from build123d import *
from build123d.topology import SkipClean

# Parameters (mm, degrees)
SKETCH1_R           = 7
SKETCH1_R_2         = 5.2
BOSS_EXTRUDE1_DEPTH = 15.66
BOSS_EXTRUDE2_START = -4
SKETCH2_W           = 6
SKETCH2_H           = 4
BOSS_EXTRUDE2_DEPTH = 4
CUT_EXTRUDE2_START  = -2
SKETCH2_3_W         = 6
SKETCH2_3_H         = 4
CUT_EXTRUDE2_DEPTH  = 2
SKETCH4_R           = 1.5
CUT_EXTRUDE1_DEPTH  = 10
FILLET7_R           = 3
BOSS_EXTRUDE3_START = -1
SKETCH5_R           = 5.2
BOSS_EXTRUDE3_DEPTH = 1
CUT_EXTRUDE3_DEPTH  = 15.66
FILLET8_R           = 3
BOSS_EXTRUDE4_DEPTH = 2


with BuildPart() as part:
    # Sketch1 → Boss-Extrude1 (new body)
    with BuildSketch(Plane(origin=(0, 0, 0), x_dir=(1, 0, 0), z_dir=(0, 1, 0))):
        with Locations(Location((0, 0, 0), (0, 0, 270))):
            Circle(SKETCH1_R)
        with Locations(Location((0, 0, 0), (0, 0, 270))):
            Circle(SKETCH1_R_2, mode=Mode.SUBTRACT)
    extrude(amount=BOSS_EXTRUDE1_DEPTH)

    # Sketch2 → Boss-Extrude2 (add)
    with BuildSketch(Plane(origin=(0, 15.66, 0), x_dir=(1, 0, 0), z_dir=(0, 1, 0)).offset(BOSS_EXTRUDE2_START)):
        with Locations((-10.67, -9)):
            Rectangle(SKETCH2_W, SKETCH2_H)
        with BuildLine():
            ThreePointArc((0, -7), (-7, 0), (0, 7))
            Line((0, 7), (-7.67, 7))
            Line((-7.67, 7), (-13.67, 7))
            Line((-13.67, 7), (-13.67, -7))
            Line((-13.67, -7), (-7.67, -7))
            Line((-7.67, -7), (0, -7))
        make_face()
        with Locations((-10.67, 9)):
            Rectangle(SKETCH2_W, SKETCH2_H)
    extrude(amount=BOSS_EXTRUDE2_DEPTH)

    # Sketch2<3> → Cut-Extrude2 (cut)
    with SkipClean():  # the faces are left unmerged after this step: merging them gives an invalid solid
        with BuildSketch(Plane(origin=(0, 15.66, 0), x_dir=(1, 0, 0), z_dir=(0, 1, 0)).offset(CUT_EXTRUDE2_START)):
            with BuildLine():
                ThreePointArc((0, -7), (-7, 0), (0, 7))
                Line((0, 7), (-7.67, 7))
                Line((-7.67, 7), (-13.67, 7))
                Line((-13.67, 7), (-13.67, -7))
                Line((-13.67, -7), (-7.67, -7))
                Line((-7.67, -7), (0, -7))
            make_face()
            with Locations((-10.67, 9)):
                Rectangle(SKETCH2_3_W, SKETCH2_3_H)
            with Locations((-10.67, -9)):
                Rectangle(SKETCH2_3_W, SKETCH2_3_H)
        extrude(amount=CUT_EXTRUDE2_DEPTH, mode=Mode.SUBTRACT)

    # Sketch4 → Cut-Extrude1 (cut)
    with SkipClean():  # the faces are left unmerged after this step: merging them gives an invalid solid
        with BuildSketch(Plane.XZ.offset(-11.66)):
            with Locations(Location((-10.68, -8, 0), (0, 0, 270))):
                Circle(SKETCH4_R)
            with Locations(Location((-10.68, 8, 0), (0, 0, 270))):
                Circle(SKETCH4_R)
        extrude(amount=-CUT_EXTRUDE1_DEPTH, mode=Mode.SUBTRACT)

    # Fillet7
    fillet7_edges = [part.edges().sort_by_distance(p)[0] for p in [
        (-7.67, 12.66, 7),
    ]]
    fillet(fillet7_edges, radius=FILLET7_R)

    # Sketch5 → Boss-Extrude3 (add)
    with SkipClean():  # the faces are left unmerged after this step: merging them gives an invalid solid
        with BuildSketch(Plane(origin=(0, 15.66, 0), x_dir=(1, 0, 0), z_dir=(0, 1, 0)).offset(BOSS_EXTRUDE3_START)):
            with Locations(Location((0, 0, 0), (0, 0, 270))):
                Circle(SKETCH5_R)
        extrude(amount=BOSS_EXTRUDE3_DEPTH)

    # Sketch6 → Cut-Extrude3 (cut)
    with BuildSketch(Plane.XZ):
        with BuildLine():
            Line((6, -3.605551275), (6, 3.605551275))
            ThreePointArc((6, 3.605551275), (7, 0), (6, -3.605551275))
        make_face()
    extrude(amount=-CUT_EXTRUDE3_DEPTH, mode=Mode.SUBTRACT)

    # Fillet8
    fillet8_edges = [part.edges().sort_by_distance(p)[0] for p in [
        (6, 15.66, 0),
    ]]
    fillet(fillet8_edges, radius=FILLET8_R)

    # Sketch7 → Boss-Extrude4 (add)
    with BuildSketch(Plane(origin=(0, 13.66, 0), x_dir=(1, 0, 0), z_dir=(0, 1, 0))):
        with BuildLine():
            Line((-13.67, 4.5), (-13.67, -4.5))
            Line((-13.67, -4.5), (-5.361902647, -4.5))
            ThreePointArc((-5.361902647, -4.5), (-7, 0), (-5.361902647, 4.5))
            Line((-5.361902647, 4.5), (-13.67, 4.5))
        make_face()
    extrude(amount=BOSS_EXTRUDE4_DEPTH)


solid = part.part
The model under review builds one solid part; all positions refer to its coordinate system, in mm. A direction names the side the tool comes from. Give positions to 0.01 mm unless a question says otherwise; leave off trailing zeros. Loops run counter-clockwise (first coordinate to the right, second up) from the corner with the lowest first, then second, coordinate; pieces in that order, holes last. Notation, with made-up numbers: (84, -13) -> (134, -13) arc R17 cw to (134, 5) -> close; hole circle Ø11 at (37, -20.5). An arc over 180 degrees is marked (long way). Put each result on its own line as item: value. Start each with the question number.
1. We need section C-C on y = 14.25. State the section outline as (x, z) points.
2. We need section B-B on z = -8. State the section outline as (x, y) points.
3. Wall thickness on probe 1 along X at (y, z) = (11.25, 0); probe 2 along Z at (x, y) = (-10.68, 12.2); probe 3 along Y at (x, z) = (1, 0.5): over which ranges is each line inside the solid? List them lowest first.
4. We need section A-A on x = -10.68. State the section outline as (y, z) points, then the cut area to 3 significant figures.
5. For faces 1 (the face through (-7.67, 13, -9)), 2 (the face through (-10, 13.66, -6)), 3 (the face through (-2, 13, 7)), list the 3-axis set-ups (+Z, -Z, +X, -X, +Y, -Y) from which the entire face can be reached by the end or side of a thin tool; tool diameter is ignored.
6. We need section D-D on z = 0. State the section outline as (x, y) points.
7. Clearance check with flat-ended pins moving along their axes: P1, Ø1.6, axis at x = -3, y = 12.5, coming from the -Z side; P2, Ø8, axis at x = -9, y = 4, coming from the -Z side; P3, Ø1.6, axis at x = -9.5, y = 14.5, coming from the -Z side. State where each tip first meets the part, or that it passes through.
8. Mouldability with a two-part tool opening along Z and no side actions: class faces 4 (the face through (-4, 13, -7)), 5 (the face through (0, 14.66, 0)), 6 (the face through (-6.81, 12.67, 7.9)) as released by +Z, released by -Z, zero draft, split by the parting line, or undercut.
Determined:
1. outline: (-13.67, -4.5) -> (-5.36, -4.5) arc R7 ccw to (5.54, -4.27) -> (5.54, 4.27) arc R7 ccw to (-5.36, 4.5) -> (-13.67, 4.5) -> close; hole circle Ø10.4 at (0, 0)
2. outline: (-13.67, 11.66) -> (-12.18, 11.66) -> (-12.18, 13.66) -> (-13.67, 13.66) -> close; (-9.18, 11.66) -> (-7.67, 11.66) -> (-7.67, 13.66) -> (-9.18, 13.66) -> close
3. probe 1: -7 to -5.2, 5.2 to 6
3. probe 2: -11 to -9.5, -6.5 to 6.5, 9.5 to 11
3. probe 3: 14.66 to 15.66
4. outline: (11.66, -11) -> (13.66, -11) -> (13.66, -9.5) -> (11.66, -9.5) -> close; (11.66, -6.5) -> (13.66, -6.5) -> (13.66, -4.5) -> (15.66, -4.5) -> (15.66, 4.5) -> (13.66, 4.5) -> (13.66, 6.5) -> (11.66, 6.5) -> close; (11.66, 9.5) -> (13.66, 9.5) -> (13.66, 11) -> (11.66, 11) -> close
4. area: 50.0 mm^2
5. face 1: -Z, +X, +Y, -Y
5. face 2: -Z, -X, +Y
5. face 3: +Z, +X, +Y, -Y
6. outline: (-13.67, 11.66) -> (-7, 11.66) -> (-7, 0) -> (-5.2, 0) -> (-5.2, 14.66) -> (5.2, 14.66) -> (5.2, 0) -> (6, 0) -> (6, 12.66) arc R3 ccw to (3, 15.66) -> (-13.67, 15.66) -> close
7. P1: z = -7
7. P2: z = -4.9
7. P3: z = -4.5
8. face 4: released by -Z
8. face 5: undercut
8. face 6: released by +Z
